from build123d import *

# Parameters (mm, degrees)
SKETCH1_R           = 1.5
BOSS_EXTRUDE1_DEPTH = 10.5
SKETCH2_R           = 2.95
BOSS_EXTRUDE2_DEPTH = 0.9
SWEEP1_PROFILE_R    = 0.85


with BuildPart() as part:
    # Sketch1 → Boss-Extrude1 (new body)
    with BuildSketch(Plane(origin=(0, 0, 0), x_dir=(0, 0, -1), z_dir=(1, 0, 0))):
        with Locations(Location((0, 0, 0), (0, 0, 180))):
            Circle(SKETCH1_R)
    extrude(amount=BOSS_EXTRUDE1_DEPTH)

    # Sketch8 → Revolve1 (revolve)
    with BuildSketch(Plane(origin=(10.5, 0, 0), x_dir=(0, 0, -1), z_dir=(1, 0, 0))):
        with BuildLine():
            Line((1.5, 0), (-1.5, 0))
            ThreePointArc((-1.5, 0), (0, 1.5), (1.5, 0))
        make_face()
    revolve(axis=Axis((10.5, 0, -1.5), (0, 0, 1)))

    # Sketch2 → Boss-Extrude2 (add)
    with BuildSketch(Plane.ZY):
        Circle(SKETCH2_R)
    extrude(amount=BOSS_EXTRUDE2_DEPTH)

    # Sweep1: sweep along a path in Sketch3
    with BuildLine(Plane.XY) as sweep1_path:
        Line((-0.9, 0), (-20.8, 0))
    # Sweep1 profile (on start of the path) → Sweep1 (sweep)
    with BuildSketch(Plane(origin=(-0.9, 0, 0), x_dir=(0, -1, 0), z_dir=(-1, 0, 0))):
        Circle(SWEEP1_PROFILE_R)
    sweep(path=sweep1_path.line)


solid = part.part
Read the model definition and answer for the solid it produces. Units are mm, in the model's axes. A direction names the side the tool comes from. Round coordinates to 2 decimals unless told otherwise and drop trailing zeros. Order: outer loops, then holes, each group sorted by start corner. A loop starts at its lowest first (then second) coordinate and runs counter-clockwise, first axis right, second up. Notation, with made-up numbers: (43.5, 74.5) - (61.5, 74.5) arc R34 cw to (61.5, 110.5) - close; hole circle Ø4 at (-19.5, -40). An arc over 180 degrees is marked (long way). Use one line per item in the form item = value. Start each with the question number.
(1) Flat-ended cylindrical pins translate along their axes: pin 1 Ø2 at (x, z) = (-8.5, 0) entering from -Y; pin 2 Ø3 at (y, z) = (-2, 0.5) entering from +X; pin 3 Ø2 at (x, y) = (-4.5, 1.5) entering from +Z. Find the tip coordinate at first contact, or state that the pin passes through.
(2) Find the intervals of material crossed by line 1 along Z through (x, y) = (-5.5, -0.1); line 2 along X through (y, z) = (0.95, 1.8); line 3 along Y through (x, z) = (-13, 0.5), in increasing order. Write a range as from..to.
(3) The part is cut by section D-D (x = 6.5). Give the vertices of the cut face in (y, z).
(4) The part is cut by section A-A (z = 0). Give the vertices of the cut face in (x, y).
(5) The part is cut by section C-C (x = -6.5). Give the vertices of the cut face in (y, z), then the cut area to 3 significant figures.
(6) For faces 1 (the face through (5.18, -0.45, 1.43)), 2 (the face through (-0.9, -1, 1)), 3 (the face through (-20.8, 0, 0)), determine the directions among +Z, -Z, +X, -X, +Y, -Y from which every point of the face is accessible in a straight line to the end or side of a thin tool.
Checked values:
q1.pin_1 = -0.85
q1.pin_2 = 11.89
q1.pin_3 = 0.69
q2.line_1 = -0.84..0.84
q2.line_2 = -0.9..0
q2.line_3 = -0.69..0.69
q3.outline = circle Ø3 at (0, 0)
q4.outline = (-20.8, -0.85) - (-0.9, -0.85) - (-0.9, -2.95) - (0, -2.95) - (0, -1.5) - (10.5, -1.5) arc R1.5 ccw to (10.5, 1.5) - (0, 1.5) - (0, 2.95) - (-0.9, 2.95) - (-0.9, 0.85) - (-20.8, 0.85) - close
q5.outline = circle Ø1.7 at (0, 0)
q5.area = 2.27 mm^2
q6.face_1 = +X
q6.face_2 = -X
q6.face_3 = +Z, -Z, -X, +Y, -Y
